Check sheet for the modelled part. Datum: model origin and axes. Units: mm. A direction names the side the tool comes from. Coordinates: 2 decimals unless noted, no trailing zeros. Order: outer loops, then holes, each group sorted by start corner. A loop starts at its lowest first (then second) coordinate and runs counter-clockwise, first axis right, second up.
1. Gauge pin test, flat ends, axial feed: pin 1 Ø1 at (y, z) = (0.5, -18) entering from -X; pin 2 Ø1.2 at (x, z) = (-11.5, 17.5) entering from +Y; pin 3 Ø0.9 at (x, z) = (-12.5, -18.5) entering from -Y. Record the tip position at first contact, or that the pin passes through.
2. Thickness scan on line 1 (Y direction, x = -17.5, z = -18); line 2 (Z direction, x = 9, y = 1.75); line 3 (Z direction, x = -14.5, y = 2.25). Record the ranges inside material, lowest first.
3. Draft check along X on faces 5 (the flat face through (-8, 9, -8)), 6 (the flat face through (12, 0, -18)), 7 (the cylindrical face through (19.48, 1.67, 18.69)). Enter one of: released by +X, released by -X, zero draft, split by the parting line, or undercut.
4. Cross-section at B-B (z = 8.15). Enter the section's corners in (x, y).
5. Set-up check for faces 1 (the flat face through (12, 0, 18)), 2 (the flat face through (-12, 0.5, 17)), 3 (the flat face through (20, 2, 0)), 4 (the flat face through (-12, 2.7, -18)): record each of +Z, -Z, +X, -X, +Y, -Y from which the full face is reachable in a straight line by a thin tool's end or side.
6. Cross-section at A-A (y = 5). Enter the section's corners in (x, z), then the cut area to 3 significant figures.
7. Cross-section at C-C (z = 1). Enter the section's corners in (x, y), then the cut area to 3 significant figures.
Autodesk Inventor part; units mm, degrees
ref_plane "Arbeitsebene1" through (-17, 4, 20) normal (1, 0, 0) x (0, -1, 0)
ref_plane "YZ Plane" through (0, 0, 0) normal (1, 0, 0) x (0, 1, 0)
ref_plane "XZ Plane" through (0, 0, 0) normal (0, 1, 0) x (-1, 0, 0)
sketch "Sketch1" plane through (0, 0, 0) normal (0, 1, 0) x (-1, 0, 0)
  line L0 (20, 20) -> (-20, 20)
  line L1 (-20, 20) -> (-20, -20)
  line L2 (-20, -20) -> (20, -20)
  line L3 (20, -20) -> (20, 20)
  circle A0 centre (10.5, 10.5) radius 4.25
  circle A1 centre (10.5, -10.5) radius 4.25
  circle A2 centre (-10.5, -10.5) radius 4.25
  circle A3 centre (-10.5, 10.5) radius 4.25
  line L4 (20, 0) -> (-20, 0) construction
  line L5 (0, 20) -> (0, -20) construction
  point P0 (0, 0)
  dimension "d0" = 40
  dimension "d1" = 40
  dimension "d2" = 8.5
  dimension "d3" = 21
  dimension "d4" = 21
extrude "Extrusion2" add sketch "Sketch1" along normal blind 2 contours L3 L2 L1 L0 | A0 | A1 | A2 | A3
sketch "Sketch2" plane through (0, 0, 0) normal (0, -1, 0) x (1, 0, 0)
  line L0 (20, 20) -> (20, -20)
  line L1 (-20, 20) -> (20, 20)
  line L2 (-20, -20) -> (-20, 20)
  line L3 (20, -20) -> (-20, -20)
  point P0 (0, 0)
extrude "Extrusion3" add sketch "Sketch2" along normal blind 0.6
sketch "Sketch3" plane through (0, 2, 0) normal (0, 1, 0) x (1, 0, 0)
  line L0 (-20, 20) -> (-20, -20)
  line L1 (-20, -20) -> (20, -20)
  line L2 (20, -20) -> (20, 20)
  line L3 (20, 20) -> (-20, 20)
  point P0 (0, 0)
extrude "Extrusion4" add sketch "Sketch3" along normal blind 2
fillet "Fillet1" radius 3 4 edges at (-20, 1.7, 20) (-20, 1.7, -20) (20, 1.7, 20) (20, 1.7, -20)
ref_plane "Arbeitsebene1" through (-17, 4, 20) normal (1, 0, 0) x (0, -1, 0)
sketch "Skizze5" plane through (-17, 4, 20) normal (1, 0, 0) x (0, -1, 0)
  line L0 (0, 0) -> (4.6, 0) construction
  line L1 (0, 0) -> (0, 3) construction
  line L2 (0.7, 0) -> (3.5, 0) construction
  line L3 (6.1491, 20) -> (-1.642, 20) construction
  line L4 (0, 40) -> (4.6, 40) construction
  line L5 (0.7, 40) -> (3.5, 40) construction
  line L6 (2.3, 0) -> (2.3, 4.6722) construction
  ellipse E0 centre (2.3, 0) end of major axis (3.5, 0) minor radius 1
  line L7 (1.1, 0) -> (3.5, 0)
  line L8 (0, 40) -> (4.6, 40) construction
  line L9 (0.7, 40) -> (3.5, 40) construction
  ellipse E1 centre (2.3, 40) end of major axis (3.5, 40) minor radius 1
  line L10 (1.1, 40) -> (3.5, 40)
  point P0 (4, 20)
  point P1 (2.3, 1)
  dimension "d22" = 2.3
  dimension "d23" = 1.2
  dimension "d28" = 1
extrude "Extrusion7" cut sketch "Skizze5" along normal blind 37 and the other way blind 5 contours L7 E0 | E1 L10 picked at (2.3176, 0.333) picked at (2.2824, 39.667)
sketch "Skizze6" plane through (0, -0.6, 0) normal (0, -1, 0) x (1, 0, 0)
  line L0 (17, 20) -> (-17, 20)
  line L1 (-20, 17) -> (-20, -17) construction
  line L2 (-14, 20) -> (-14, 16.5)
  line L3 (-14, 20) -> (-10, 20)
  line L4 (0, 16.6905) -> (0, 25.5183)
  line L5 (7.2129, 0) -> (-7.9382, 0)
  line L6 (-17, 20) -> (17, 20)
  line L7 (14, 20) -> (10, 20)
  line L8 (17, -20) -> (-17, -20)
  line L9 (-14, 16.5) -> (-10, 16.5)
  line L10 (-10, 16.5) -> (-10, 20)
  line L11 (-17, -20) -> (17, -20)
  line L12 (14, 20) -> (14, 16.5)
  line L13 (14, 16.5) -> (10, 16.5)
  line L14 (10, 16.5) -> (10, 20)
  line L15 (-14, -20) -> (-14, -16.5)
  line L16 (-14, -16.5) -> (-10, -16.5)
  line L17 (-10, -16.5) -> (-10, -20)
  line L18 (10, -16.5) -> (10, -20)
  line L19 (14, -16.5) -> (10, -16.5)
  line L20 (14, -20) -> (14, -16.5)
  point P0 (0, 0)
  point P1 (-12, 20)
  dimension "d34" = 8
  dimension "d35" = 2
  dimension "d41" = 3.5
  dimension "d42" = 4
extrude "Extrusion8" cut sketch "Skizze6" against normal blind 3.3
sketch "Skizze8" plane through (0, -0.6, 0) normal (0, -1, 0) x (1, 0, 0)
  line L0 (-10, 20) -> (-10, 16.5)
  line L1 (-10, 16.5) -> (-14, 16.5)
  line L2 (-14, -20) -> (-14, -16.5)
  line L3 (-14, -16.5) -> (-10, -16.5)
  line L4 (-10, -16.5) -> (-10, -20)
  line L5 (-10, -20) -> (10, -20)
  line L6 (10, -20) -> (10, -16.5)
  line L7 (10, -16.5) -> (14, -16.5)
  line L8 (14, -16.5) -> (14, -20)
  line L9 (14, -20) -> (17, -20)
  arc A0 (17, -20) -> (20, -17) centre (17, -17) ccw
  line L10 (20, -17) -> (20, 17)
  arc A1 (20, 17) -> (17, 20) centre (17, 17) ccw
  line L11 (17, 20) -> (14, 20)
  line L12 (14, 20) -> (14, 16.5)
  line L13 (14, 16.5) -> (10, 16.5)
  line L14 (10, 16.5) -> (10, 20)
  line L15 (10, 20) -> (-10, 20)
  line L16 (-10, 20) -> (-10, 16.5)
  line L17 (-10, 16.5) -> (-14, 16.5)
  line L18 (-14, 16.5) -> (-14, 20)
  line L19 (-14, 20) -> (-17, 20)
  arc A2 (-17, 20) -> (-20, 17) centre (-17, 17) ccw
  line L20 (-20, 17) -> (-20, -17)
  arc A3 (-20, -17) -> (-17, -20) centre (-17, -17) ccw
  line L21 (-17, -20) -> (-14, -20)
  line L22 (0, 16.7549) -> (0, 9.0333)
  line L23 (12, 0) -> (-14, 0)
  line L24 (-10, 16.5) -> (-14, 16.5)
  line L25 (-14, 16.5) -> (-14, 18)
  line L26 (-14, 18) -> (-10, 18)
  line L27 (-10, 18) -> (-10, 16.5)
  line L28 (10, 20) -> (10, 16.5)
  line L29 (10, 16.5) -> (14, 16.5)
  line L30 (14, 16.5) -> (14, 18)
  line L31 (14, 18) -> (10, 18)
  line L32 (10, 18) -> (10, 16.5)
  line L33 (-14, -18) -> (-10, -18)
  line L34 (14, -18) -> (10, -18)
  point P0 (0, 0)
  dimension "d47" = 1.5
extrude "Extrusion10" add sketch "Skizze8" against normal blind 1.1 contours L0 L1 L18 L26 | L31 L12 L13 L14 | L2 L3 L4 L33 | L34 L6 L7 L8
sketch "Skizze9" plane through (0, 4, 0) normal (0, 1, 0) x (1, 0, 0)
  line L0 (-20, 17) -> (-20, -17)
  circle A0 centre (-8, -8.15) radius 1.4
  line L1 (-2.4635, 0) -> (-12.5282, 0) construction
  circle A1 centre (-8, 8.15) radius 1.4
  point P0 (0, 0)
  dimension "d55" = 8.15
  dimension "d56" = 12
  dimension "d57" = 2.8
extrude "Extrusion11" add sketch "Skizze9" along normal blind 5
chamfer "Fasen2" distance 0.5 angle 45 2 edges at (-9.4, 4, -8.15) (-9.4, 4, 8.15)
properties part number "IMU_mount_baseplate"
Data:
1. pin 1: stops at x = -19.96
1. pin 2: stops at y = 4
1. pin 3: stops at y = 2.7
2. line 1: y = -0.6 to 4
2. line 2: z = -19 to 19
2. line 3: z = -19.11 to 19.11
3. face 5: zero draft
3. face 6: undercut
3. face 7: released by +X
4. outline: (-20, -0.6) - (20, -0.6) - (20, 4) - (-6.1, 4) - (-6.6, 4.5) - (-6.6, 9) - (-9.4, 9) - (-9.4, 4.5) - (-9.9, 4) - (-20, 4) - close
5. face 1: +Z, -Y
5. face 2: +Z
5. face 3: +Z, -Z, +X, +Y, -Y
5. face 4: -Z
6. outline: circle Ø2.8 at (-8, -8.15); circle Ø2.8 at (-8, 8.15)
6. area: 12.3 mm2
7. outline: (-20, -0.6) - (20, -0.6) - (20, 4) - (-20, 4) - close
7. area: 184 mm2
